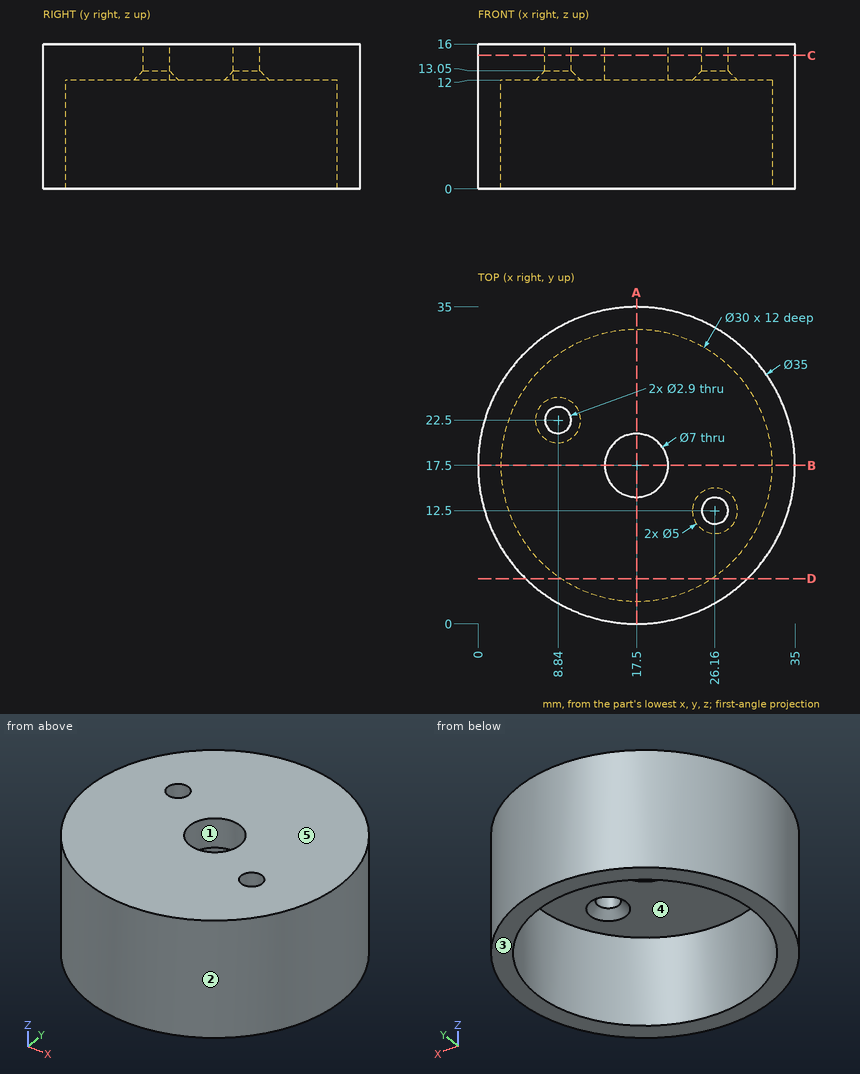
Source: three-view drawing plus pictorial views. Frame: mm from the lowest corner of the part. A direction names the side the tool comes from. Give positions to 0.01 mm unless a question says otherwise; leave off trailing zeros. Order: outer loops, then holes, each group sorted by start corner. A loop starts at its lowest first (then second) coordinate and runs counter-clockwise, first axis right, second up.
1. Mould query, pull axis X, two halves, no side actions, for the marked faces 1, 2 and 3. Classes: released by +X, released by -X, zero draft, split by the parting line, or undercut.
Derived:
face 1: undercut
face 2: split by the parting line
face 3: zero draft
2. Section D-D on y = 5. Return the cut outline in (x, z).
Derived:
outline: (5.25, 0) - (9.21, 0) - (9.21, 12) - (25.79, 12) - (25.79, 0) - (29.75, 0) - (29.75, 16) - (5.25, 16) - close
3. Reachability of the marked faces 4 and 5 from +Z, -Z, +X, -X, +Y, -Y: full face, straight path, thin tool, end or side. Return the list, or none.
Derived:
face 4: -Z
face 5: +Z, +X, -X, +Y, -Y
4. Pin query (flat end, axial travel): pin 1 (11 mm diameter, centred on x = 17.5, y = 17.5, fed in from -Z); pin 2 (1.5 mm diameter, centred on x = 7.5, z = 7.5, fed in from -Y) (1 decimal); pin 3 (2 mm diameter, centred on y = 11, z = 12.5, fed in from +X); pin 4 (2.5 mm diameter, centred on x = 26.16, y = 12.5, fed in from +Z). Return the tip coordinate at first contact, or that it passes through.
Derived:
pin 1: stops at z = 12
pin 2: stops at y = 2.6
pin 3: stops at x = 34.11
pin 4: passes through
5. Section A-A on x = 17.5. Return the cut outline in (y, z).
Derived:
outline: (0, 0) - (2.5, 0) - (2.5, 12) - (14, 12) - (14, 16) - (0, 16) - close; (21, 12) - (32.5, 12) - (32.5, 0) - (35, 0) - (35, 16) - (21, 16) - close
6. Material intervals for L1, parallel to Y at x = 18, z = 4.5; L2, parallel to Y at x = 21, z = 10.5; L3, parallel to X at y = 5, z = 7, sorted ascending.
Derived:
L1: y = 0.01 to 2.51, 32.49 to 34.99
L2: y = 0.35 to 2.91, 32.09 to 34.65
L3: x = 5.25 to 9.21, 25.79 to 29.75
7. Section C-C on z = 14.75. Return the cut outline in (x, y), and give its area (3 significant figures).
Derived:
outline: circle Ø35 at (17.5, 17.5); hole circle Ø2.9 at (8.84, 22.5); hole circle Ø7 at (17.5, 17.5); hole circle Ø2.9 at (26.16, 12.5)
area: 910 mm2
